Could you check a few things on this drawing? It's one solid part, dimensions in mm from its lowest x, y, z. A direction names the side the tool comes from. Coordinates: 2 decimals unless noted, no trailing zeros. Loops run counter-clockwise (first coordinate to the right, second up) from the corner with the lowest first, then second, coordinate; pieces in that order, holes last. Notation, with made-up numbers: M 68,-24.75 L 84,-24.75 A31 cw 84,7.25 Z; hole C 11.5,-8.75 d11. An arc over 180 degrees is marked long. Answer as a JSON object with one key per item and string values. Group by question number.
Item 1: Which directions (+Z, -Z, +X, -X, +Y, -Y) give clear straight access to the entire face, cutting with the end or side of a thin tool? Please do the marked faces 5 and 6.
Item 2: Suppose I cut it at A-A (x = 15). Write out the boundary of the cut face in (y, z) (1 decimal).
Item 3: Suppose I cut it at C-C (z = 0.75). Write out the boundary of the cut face in (x, y) (1 decimal).
Item 4: We'd pull the mould along X, two halves only. Please class the marked faces 1, 2, 3 and 4: +X half, -X half, draft (parallel to the pull), parting line (faces both ways), or undercut.
Item 5: I'm going to push flat-ended pins straight in: pin 1 Ø2.5 at (x, y) = (23.25, 10.24) entering from -Z; pin 2 Ø1.5 at (x, z) = (14, 2.5) entering from +Y; pin 3 Ø1 at (y, z) = (19, 5) entering from -X. Where does each tip first touch, or does it pass through?
Item 6: If I drill on line 1 (Y direction, x = 15, z = 3.75) (1 decimal); line 2 (X direction, y = 10, z = 2.5) (1 decimal); line 3 (Z direction, x = 18.5, y = 2.25), over which ranges is the centre line in solid material (lowest first)?
Item 7: Suppose I cut it at B-B (y = 15). Write out the boundary of the cut face in (x, z), then the cut area to 3 significant figures.
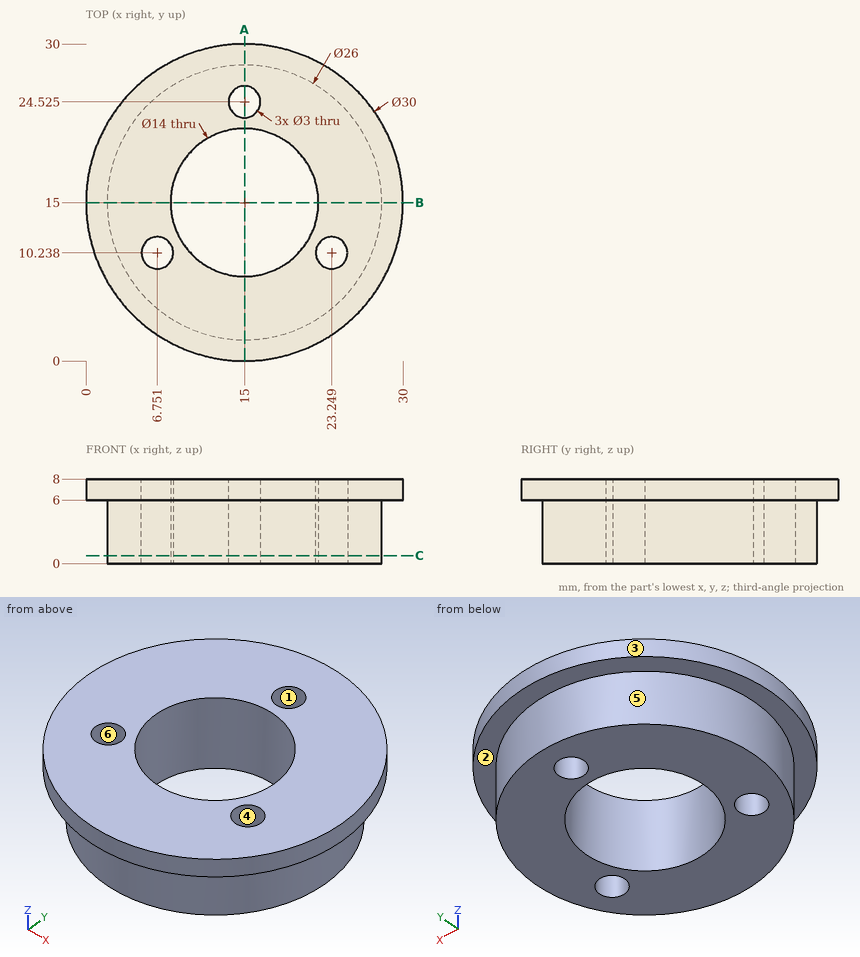
From the geometry:
{
 "1": {"face 5": "-Z", "face 6": "+Z, -Z"},
 "2": {"outline": "M 0,6 L 2,6 L 2,0 L 8,0 L 8,8 L 0,8 Z; M 22,0 L 23,0 L 23,8 L 22,8 Z; M 26,0 L 28,0 L 28,6 L 30,6 L 30,8 L 26,8 Z"},
 "3": {"outline": "C 15,15 d26; hole C 6.8,10.2 d3; hole C 15,15 d14; hole C 15,24.5 d3; hole C 23.2,10.2 d3"},
 "4": {"face 1": "undercut", "face 2": "draft", "face 3": "parting line", "face 4": "undercut"},
 "5": {"pin 1": "through", "pin 2": "y = 28", "pin 3": "x = 2.48"},
 "6": {"line 1": "2 to 8, 22 to 23, 26 to 28", "line 2": "3 to 5.3, 8.2 to 10.1, 19.9 to 21.8, 24.7 to 27", "line 3": "6 to 8"},
 "7": {"outline": "M 0,6 L 2,6 L 2,0 L 8,0 L 8,8 L 0,8 Z; M 22,0 L 28,0 L 28,6 L 30,6 L 30,8 L 22,8 Z", "area": "104 mm2"}
}
